```python
from build123d import *

# Parameters (mm, degrees)
SALIENTE_EXTRUIR1_DEPTH = 9
CROQUIS2_R              = 14.5
CORTAR_EXTRUIR1_DEPTH   = 28
REDONDEO1_R             = 1
CROQUIS4_R              = 24
SALIENTE_EXTRUIR2_DEPTH = 5
CROQUIS5_R              = 14.5
CORTAR_EXTRUIR2_DEPTH   = 35.307433597
REDONDEO2_R             = 2
VACIADO1_OUTLINE_R      = 23
VACIADO1_OUTLINE_R_2    = 15.5
VACIADO1_DEPTH          = 2.9999999
VACIADO1_2_OUTLINE_R    = 15.5
VACIADO1_2_DEPTH        = 8


with BuildPart() as part:
    # Croquis1 → Saliente-Extruir1 (new body)
    with BuildSketch(Plane(origin=(0, 0, 0), x_dir=(1, 0, 0), z_dir=(0, 1, 0))):
        Polygon((18, 7.455844123), (7.455844123, 18), (-7.455844123, 18), (-18, 7.455844123), (-18, -7.455844123), (-7.455844123, -18), (7.455844123, -18), (18, -7.455844123), align=None)
    extrude(amount=SALIENTE_EXTRUIR1_DEPTH)

    # Croquis2 → Cortar-Extruir1 (cut, through all)
    with BuildSketch(Plane(origin=(0, 9, 0), x_dir=(1, 0, 0), z_dir=(0, 1, 0))):
        with Locations(Location((0, 0, 0), (0, 0, 270))):
            Circle(CROQUIS2_R)
    extrude(amount=-CORTAR_EXTRUIR1_DEPTH, mode=Mode.SUBTRACT)

    # Redondeo1
    redondeo1_edges = [part.edges().sort_by_distance(p)[0] for p in [
        (0, 9, -18),
        (-12.727922061, 9, -12.727922061),
        (-18, 9, 0),
        (-12.727922061, 9, 12.727922061),
        (0, 9, 18),
        (12.727922061, 9, 12.727922061),
        (18, 9, 0),
        (12.727922061, 9, -12.727922061),
    ]]
    fillet(redondeo1_edges, radius=REDONDEO1_R)

    # Croquis4 → Saliente-Extruir2 (add)
    with BuildSketch(Plane(origin=(0, 5, 0), x_dir=(1, 0, 0), z_dir=(0, 1, 0))):
        with Locations(Location((0, 0, 0), (0, 0, 270))):
            Circle(CROQUIS4_R)
    extrude(amount=-SALIENTE_EXTRUIR2_DEPTH)

    # Croquis5 → Cortar-Extruir2 (cut, through all)
    with BuildSketch(Plane(origin=(0, 5, 0), x_dir=(1, 0, 0), z_dir=(0, 1, 0))):
        with Locations(Location((0, 0, 0), (0, 0, 270))):
            Circle(CROQUIS5_R)
    extrude(amount=-CORTAR_EXTRUIR2_DEPTH, mode=Mode.SUBTRACT)

    # Redondeo2
    redondeo2_edges = [part.edges().sort_by_distance(p)[0] for p in [
        (0, 5, -24),
    ]]
    fillet(redondeo2_edges, radius=REDONDEO2_R)

    # Vaciado1: read off the stored shape, not the designer's step
    # Vaciado1 outline → Vaciado1 (cut)
    with BuildSketch(Plane(origin=(0, 0, 0), x_dir=(1, 0, 0), z_dir=(0, 1, 0))):
        Circle(VACIADO1_OUTLINE_R)
        Circle(VACIADO1_OUTLINE_R_2, mode=Mode.SUBTRACT)
    extrude(amount=VACIADO1_DEPTH, mode=Mode.SUBTRACT)

    # Vaciado1 2 outline → Vaciado1 2 (cut)
    with BuildSketch(Plane(origin=(0, 0, 0), x_dir=(1, 0, 0), z_dir=(0, 1, 0))):
        Polygon((17, -7.04163056), (17, 7.04163056), (7.04163056, 17), (-7.04163056, 17), (-17, 7.04163056), (-17, -7.04163056), (-7.04163056, -17), (7.04163056, -17), align=None)
        Circle(VACIADO1_2_OUTLINE_R, mode=Mode.SUBTRACT)
    extrude(amount=VACIADO1_2_DEPTH, mode=Mode.SUBTRACT)

    # Vaciado1 3 outline → Vaciado1 3 (revolve, cut)
    with BuildSketch(Plane.XY):
        with BuildLine():
            Line((17, 2.9999999), (23, 3))
            ThreePointArc((23, 3), (22.707106781, 3.707106781), (22, 4))
            Line((22, 4), (17, 4))
            Line((17, 4), (17, 2.9999999))
        make_face()
    revolve(axis=Axis((0, 0, 0), (0, 1, 0)), mode=Mode.SUBTRACT)


solid = part.part
```
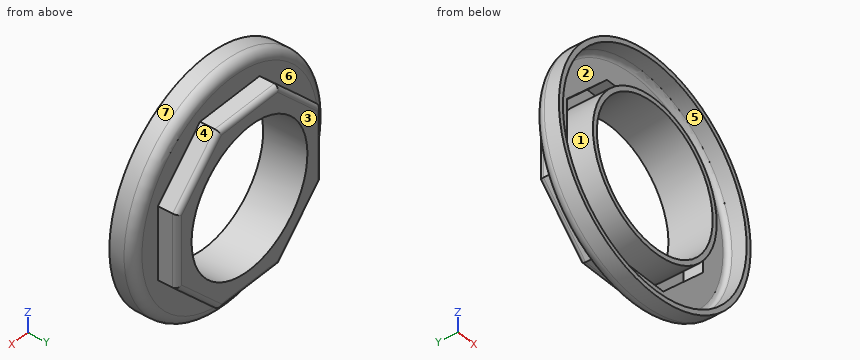
Geometry check sheet. Reference: the model listing, model coordinates, mm. Face numbers are marked on the shaded views. A direction names the side the tool comes from. Round coordinates to 2 decimals unless told otherwise and drop trailing zeros. Order: outer loops, then holes, each group sorted by start corner. A loop starts at its lowest first (then second) coordinate and runs counter-clockwise, first axis right, second up. Notation, with made-up numbers: M 61,79.5 L 90,79.5 A7 ccw 90,83.5 Z; hole C -6.5,-33 d10. An arc over 180 degrees is marked long. Write item = value, one per line.
Q1. Release check for a two-part mould opening along X. For the marked faces 1, 2, 3 and 4 record: released by +X, released by -X, zero draft, split by the parting line, or undercut.
Answer block:
face_1 = undercut
face_2 = undercut
face_3 = zero draft
face_4 = released by +X
Q2. Depth check by flat-ended pin: pin 1 Ø2.5 at (x, y) = (-3, 6.5) entering from -Z; pin 2 Ø4 at (x, y) = (13.5, 2) entering from +Z; pin 3 Ø0.9 at (x, y) = (-2, 6.5) entering from +Z; pin 4 Ø12 at (x, z) = (13, 6) entering from +Y. Enter the tip coordinate at first touch or a pass-through.
Answer block:
pin_1 = -18
pin_2 = 21.07
pin_3 = 18
pin_4 = 9
Q3. Section check B-B (y = 6.5). Enter the section's corners in (x, z).
Answer block:
outline = M -18,-7.46 L -7.46,-18 L 7.46,-18 L 18,-7.46 L 18,7.46 L 7.46,18 L -7.46,18 L -18,7.46 Z; C 0,0 d31; hole M -17,-7.04 L -7.04,-17 L 7.04,-17 L 17,-7.04 L 17,7.04 L 7.04,17 L -7.04,17 L -17,7.04 Z; hole C 0,0 d29
Q4. Section check D-D (y = 1.5). Enter the section's corners in (x, z), plus the area to 3 significant figures.
Answer block:
outline = C 0,0 d48; C 0,0 d31; hole C 0,0 d46; hole C 0,0 d29
area = 242 mm^2
Q5. Scan lines: line 1 (X direction, y = 5.75, z = 0); line 2 (X direction, y = 6, z = -2); line 3 (Z direction, x = -5, y = 6.25). Record each from-to range of solid material in increasing order.
Answer block:
line_1 = -18 to -17, -15.5 to -14.5, 14.5 to 15.5, 17 to 18
line_2 = -18 to -17, -15.37 to -14.36, 14.36 to 15.37, 17 to 18
line_3 = -18 to -17, -14.67 to -13.61, 13.61 to 14.67, 17 to 18
Q6. Set-up check for the marked faces 5, 6 and 7: record each of +Z, -Z, +X, -X, +Y, -Y from which the full face is reachable in a straight line by a thin tool's end or side.
Answer block:
face_5 = -Y
face_6 = +Y
face_7 = +Y, -Y
